```python
from build123d import *
from build123d.topology import SkipClean

# Parameters (mm, degrees)
SKETCH_1_R      = 0.95
EXTRUDE_1_DEPTH = 2
EXTRUDE_START   = 3
SKETCH_2_W      = 8
SKETCH_2_H      = 5
SKETCH_2_R      = 0.95
SKETCH_2_W_2    = 13
SKETCH_2_H_2    = 3.5
EXTRUDE_2_DEPTH = 3
SKETCH_4_W      = 35
SKETCH_4_H      = 10
EXTRUDE_3_DEPTH = 2
SKETCH_5_W      = 15
SKETCH_5_H      = 20
SKETCH_5_R      = 3
EXTRUDE_4_DEPTH = 3


with BuildPart() as part:
    # 草图1 → 凸台-拉伸1 (new body)
    with BuildSketch(Plane.XY):
        Polygon((-17.5, 6.5), (-4.5, 6.5), (-4.5, 9), (17.5, 9), (17.5, -9), (-17.5, -9), align=None)
        with Locations((15, -6.35)):
            Circle(SKETCH_1_R, mode=Mode.SUBTRACT)
    extrude(amount=EXTRUDE_1_DEPTH)

    # 草图2 → 凸台-拉伸2 (add)
    # profile 1 of 2: a face of its own
    with SkipClean():  # the faces are left unmerged after this step: merging them gives an invalid solid
        with BuildSketch(Plane(origin=(0, 0, 0), x_dir=(-1, 0, 0), z_dir=(0, 0, -1)).offset(EXTRUDE_START)):
            with Locations((-13.5, -6.5)):
                Rectangle(SKETCH_2_W, SKETCH_2_H)
            with Locations((-15, -6.35)):
                Circle(SKETCH_2_R, mode=Mode.SUBTRACT)
        # profile 2 of 2: a face of its own
        with BuildSketch(Plane(origin=(0, 0, 0), x_dir=(-1, 0, 0), z_dir=(0, 0, -1)).offset(EXTRUDE_START)):
            with Locations((11, 4.75)):
                Rectangle(SKETCH_2_W_2, SKETCH_2_H_2)
        extrude(amount=-EXTRUDE_2_DEPTH)

    # 草图4 → 凸台-拉伸3 (add)
    with SkipClean():  # the faces are left unmerged after this step: merging them gives an invalid solid
        with BuildSketch(Plane.XZ.offset(9)):
            with Locations((0, -3)):
                Rectangle(SKETCH_4_W, SKETCH_4_H)
        extrude(amount=EXTRUDE_3_DEPTH)

    # 草图5 → 凸台-拉伸4 (add)
    with SkipClean():  # the faces are left unmerged after this step: merging them gives an invalid solid
        with BuildSketch(Plane(origin=(17.5, 0, 0), x_dir=(0, 0, -1), z_dir=(1, 0, 0))):
            with Locations((-4.5, -1)):
                Rectangle(SKETCH_5_W, SKETCH_5_H)
            with Locations((-7, -1)):
                Circle(SKETCH_5_R, mode=Mode.SUBTRACT)
        extrude(amount=EXTRUDE_4_DEPTH)


solid = part.part
```
Design review of the part built by this model. Coordinates are the model's own, in mm. A direction names the side the tool comes from. Give positions to 0.01 mm unless a question says otherwise; leave off trailing zeros. Loops run counter-clockwise (first coordinate to the right, second up) from the corner with the lowest first, then second, coordinate; pieces in that order, holes last. Notation, with made-up numbers: (-20, 30.25) -> (-16, 30.25) arc R26 ccw to (-16, 66.25) -> close; hole circle Ø3 at (34, 85). An arc over 180 degrees is marked (long way). Write each question's results on one line, items separated by ' | '.
Q1. Wall thickness on L1, parallel to Y at x = 18.25, z = 7; L2, parallel to X at y = -6.35, z = -2.2; L3, parallel to Z at x = 6, y = -3: over which ranges is each line inside the solid? List them lowest first.
Reply:
L1: y = -11 to -4, 2 to 9 | L2: x = 9.5 to 14.05, 15.95 to 20.5 | L3: z = 0 to 2
Q2. Take a section at A-A, the plane z = -1.5. Write out the cut boundary in (x, y), plus the area to 3 significant figures.
Reply:
outline: (-17.5, -11) -> (20.5, -11) -> (20.5, 9) -> (17.5, 9) -> (17.5, -4) -> (9.5, -4) -> (9.5, -9) -> (-17.5, -9) -> close; (-17.5, 3) -> (-4.5, 3) -> (-4.5, 6.5) -> (-17.5, 6.5) -> close; hole circle Ø1.9 at (15, -6.35) | area: 213 mm²
Q3. Take a section at B-B, the plane y = -1. Write out the cut boundary in (x, z), plus the area to 3 significant figures.
Reply:
outline: (-17.5, 0) -> (17.5, 0) -> (17.5, -3) -> (20.5, -3) -> (20.5, 4) -> (17.5, 4) -> (17.5, 2) -> (-17.5, 2) -> close; (17.5, 10) -> (20.5, 10) -> (20.5, 12) -> (17.5, 12) -> close | area: 97.0 mm²
Q4. Take a section at C-C, the plane x = -12.5. Write out the cut boundary in (y, z).
Reply:
outline: (-11, -8) -> (-9, -8) -> (-9, 0) -> (3, 0) -> (3, -3) -> (6.5, -3) -> (6.5, 2) -> (-11, 2) -> close
Q5. For pin 1 Ø5.5 at (x, y) = (-7, -3.5) entering from -Z; pin 2 Ø0.9 at (x, y) = (19.5, -1) entering from -Z; pin 3 Ø2 at (x, y) = (-8, -10) entering from +Z, all flat-tipped, find the tip position at first contact; note any pin that passes through.
Reply:
pin 1: stops at z = 0 | pin 2: stops at z = -3 | pin 3: stops at z = 2
Q6. The part is to be moulded in two halves that separate along Y. For faces 1 (the face through (18.98, -2.15, 4.23)), 2 (the face through (14, -4, -2)), 3 (the face through (9.5, -7, -2)), say which applies: +Y half, -Y half, draft (parallel to the pull), parting line (faces both ways), or undercut.
Reply:
face 1: undercut | face 2: +Y half | face 3: draft
Q7. Take a section at D-D, the plane z = 7. Write out the cut boundary in (x, y), plus the area to 3 significant figures.
Reply:
outline: (17.5, -11) -> (20.5, -11) -> (20.5, -4) -> (17.5, -4) -> close; (17.5, 2) -> (20.5, 2) -> (20.5, 9) -> (17.5, 9) -> close | area: 42.0 mm²
Q8. Machinability: for faces 4 (the face through (17.5, -10, -6)), 5 (the face through (17.5, 1.4, 9.3)), 6 (the face through (0, -9, -4)), 7 (the face through (-11, 5, -3)), 8 (the face through (17.5, 3, -1)), which of the approach directions +Z, -Z, +X, -X, +Y, -Y give a long, thin tool a straight path to every point of the face, cutting with its end or side? Answer none if there is none.
Reply:
face 4: -Z, +X, +Y, -Y | face 5: +Z, -X, +Y, -Y | face 6: -Z, -X | face 7: -Z, +X, -X, +Y | face 8: -Z, +Y
